The listing builds one solid part. Answer for the finished solid, in the listing's coordinates (mm). A direction names the side the tool comes from. Coordinates: 2 decimals unless noted, no trailing zeros. Write each loop counter-clockwise with the first axis right and the second up, starting at its lowest first coordinate (ties: lowest second). Pieces come first, ordered by that corner, then holes.
from build123d import *

# Parameters (mm, degrees)
BOSS_EXTRUDE1_DEPTH = 10
BOSS_EXTRUDE2_DEPTH = 50
SKETCH3_R           = 5
CUT_EXTRUDE1_DEPTH  = 188.082869339
SKETCH4_R           = 5
CUT_EXTRUDE2_DEPTH  = 10
SKETCH5_R           = 5
CUT_EXTRUDE3_DEPTH  = 10


with BuildPart() as part:
    # Sketch1 → Boss-Extrude1 (new body)
    with BuildSketch(Plane.XY):
        Polygon((0, 150), (50, 150), (50, 50), (100, 50), (100, 0), (0, 0), align=None)
    extrude(amount=BOSS_EXTRUDE1_DEPTH)

    # Sketch2 → Boss-Extrude2 (add)
    with BuildSketch(Plane.XY.offset(10)):
        Polygon((40, 150), (40, 40), (100, 40), (100, 50), (50, 50), (50, 150), align=None)
    extrude(amount=BOSS_EXTRUDE2_DEPTH)

    # Sketch3 → Cut-Extrude1 (cut, through all)
    with BuildSketch(Plane.XY.offset(10)):
        with Locations((20, 20)):
            Circle(SKETCH3_R)
        with Locations((20, 120)):
            Circle(SKETCH3_R)
        with Locations((20, 75)):
            Circle(SKETCH3_R)
        with Locations((70, 20)):
            Circle(SKETCH3_R)
    extrude(amount=-CUT_EXTRUDE1_DEPTH, mode=Mode.SUBTRACT)

    # Sketch4 → Cut-Extrude2 (cut)
    with BuildSketch(Plane.ZY.offset(-40)):
        with Locations(Location((35, 122.555580901, 0), (0, 0, 270))):
            Circle(SKETCH4_R)
        with Locations(Location((35, 81.685491979, 0), (0, 0, 270))):
            Circle(SKETCH4_R)
    extrude(amount=-CUT_EXTRUDE2_DEPTH, mode=Mode.SUBTRACT)

    # Sketch5 → Cut-Extrude3 (cut)
    with BuildSketch(Plane.XZ.offset(-40)):
        with Locations(Location((70, 35, 0), (0, 0, 270))):
            Circle(SKETCH5_R)
    extrude(amount=-CUT_EXTRUDE3_DEPTH, mode=Mode.SUBTRACT)


solid = part.part
Q1. Which of the six approach directions +Z, -Z, +X, -X, +Y, -Y give full straight-line access (tool end or side, diameter ignored) to faces 5 (the face through (50, 99, 30)), 6 (the face through (100, 41, 16)), 7 (the face through (70, 40, 29)), 8 (the face through (40, 96, 35)), 9 (the face through (42, 150, 16))?
Answers below:
face 5: +Z, -Z, +X, +Y
face 6: +Z, -Z, +X, +Y, -Y
face 7: +Z, +X, -X, -Y
face 8: +Z, -X, +Y, -Y
face 9: +Z, -Z, +X, -X, +Y
Q2. The part is cut by section D-D, the plane y = 55. Write down the section's boundary in (x, z).
Answers below:
outline: (0, 0) - (50, 0) - (50, 60) - (40, 60) - (40, 10) - (0, 10) - close
Q3. Given pin 1 (11.5 mm diameter, centred on y = 81.69, z = 35, fed in from +X); pin 2 (6 mm diameter, centred on y = 126.5, z = 24, fed in from -X); pin 3 (25 mm diameter, centred on x = 77, z = 31, fed in from -Y); pin 4 (2 mm diameter, centred on x = 33, y = 132, fed in from -Z), each flat-ended and moving along its own axis, determine where each tip first touches the part or whether it passes through.
Answers below:
pin 1: stops at x = 50
pin 2: stops at x = 40
pin 3: stops at y = 40
pin 4: stops at z = 0
Q4. The part is cut by section C-C, the plane z = 48. Write down the section's boundary in (x, y), then the cut area to 3 significant figures.
Answers below:
outline: (40, 40) - (100, 40) - (100, 50) - (50, 50) - (50, 150) - (40, 150) - close
area: 1,600 mm2
Q5. The part is cut by section A-A, the plane y = 75. Write down the section's boundary in (x, z).
Answers below:
outline: (0, 0) - (15, 0) - (15, 10) - (0, 10) - close; (25, 0) - (50, 0) - (50, 60) - (40, 60) - (40, 10) - (25, 10) - close
Q6. Determine the mould class of faces 1 (the face through (75, 50, 30)), 2 (the face through (18.92, 115.12, 5.07)), 3 (the face through (39.6, 59.4, 10)), 4 (the face through (44.93, 127.55, 35.22)) for opening direction Y: released by +Y, released by -Y, zero draft, split by the parting line, or undercut.
Answers below:
face 1: released by +Y
face 2: undercut
face 3: zero draft
face 4: undercut
Q7. The part is cut by section B-B, the plane x = 18.5. Write down the section's boundary in (y, z).
Answers below:
outline: (0, 0) - (15.23, 0) - (15.23, 10) - (0, 10) - close; (24.77, 0) - (70.23, 0) - (70.23, 10) - (24.77, 10) - close; (79.77, 0) - (115.23, 0) - (115.23, 10) - (79.77, 10) - close; (124.77, 0) - (150, 0) - (150, 10) - (124.77, 10) - close
Q8. Find the intervals of material crossed by probe 1 along Y at (x, z) = (20, 3.75); probe 2 along Y at (x, z) = (94, 47); probe 3 along Y at (x, z) = (49.5, 40.5), in increasing order.
Answers below:
probe 1: y = 0 to 15, 25 to 70, 80 to 115, 125 to 150
probe 2: y = 40 to 50
probe 3: y = 40 to 150
